CAD build for the part. Positions are in the model's coordinates, mm. A direction names the side the tool comes from. Round coordinates to 2 decimals unless told otherwise and drop trailing zeros. Write each loop counter-clockwise with the first axis right and the second up, starting at its lowest first coordinate (ties: lowest second). Pieces come first, ordered by that corner, then holes. Notation, with made-up numbers: (40, -25) - (82, -25) arc R12 ccw to (82, -9) - close; hole circle Ø5 at (65, 13). An arc over 180 degrees is marked (long way). Put each result on its own line as item: value. Start each with the question number.
Item 1: Mould opens along Z. For faces 1 (the flat face through (30, 1, -150)), 2 (the flat face through (-25.4, 1.48, -132.08)), 3 (the cylindrical face through (-0.88, 1.48, -122.9)) say: released by +Z, released by -Z, zero draft, split by the parting line, or undercut.
Item 2: Cut at A-A (z = -157.5). Give the cut face in (x, y), and give its area (3 significant figures).
Item 3: 3-axis set-ups, long thin cutter, end or side, ignore diameter. For faces 4 (the cylindrical face through (22.39, 1.48, -136.02)), 5 (the flat face through (-15, 1, -126.088)), 6 (the flat face through (15, 1, -126.088)): which of +Z, -Z, +X, -X, +Y, -Y reach the whole face in a straight line?
Item 4: Drill centre lines: line 1 (X direction, y = 1, z = -157.5); line 2 (X direction, y = 1.85, z = -136); line 3 (Z direction, x = -14, y = 0.8). Where is each one in solid material? Low to high. Write a range as from..to.
Item 5: Pin check, flat tips, straight feed: pin 1 Ø1 at (y, z) = (1.5, -128.5) entering from -X; pin 2 Ø4 at (x, z) = (14.1, -141.03) entering from +Y; pin 3 Ø0.9 at (y, z) = (2, -121.5) entering from -X; pin 4 Ø1.5 at (x, y) = (-14, 2) entering from +Z. Stop position of each tip, or through.
Item 6: Cut at B-B (x = 0). Give the cut face in (y, z).
Item 7: Cut at C-C (z = -141.5). Give the cut face in (x, y).
Item 8: Cut at D-D (y = 0.45). Count the separate pieces of the cut face and the enclosed holes in it, and give its area (3 significant figures).
```python
from build123d import *

# Parameters (mm, degrees)
SKETCH_1_R      = 1.45
EXTRUDE_1_DEPTH = 3
FILLET_1_R      = 3


with BuildPart() as part:
    # 草图1 → 凸台-拉伸1 (new body)
    with BuildSketch(Plane(origin=(0, 0, 0), x_dir=(1, 0, 0), z_dir=(0, 1, 0))):
        Polygon((30, 165), (-30, 165), (-30, 137.678611726), (-20.478927243, 126.087702635), (-7.5, 126.087702635), (-7.5, 116.748929431), (7.5, 116.748929431), (7.5, 126.087702635), (20.478927243, 126.087702635), (30, 137.678611726), align=None)
        with Locations(Location((0, 157.5, 0), (0, 0, 270))):
            Circle(SKETCH_1_R, mode=Mode.SUBTRACT)
        with Locations(Location((-15, 157.5, 0), (0, 0, 270))):
            Circle(SKETCH_1_R, mode=Mode.SUBTRACT)
        with Locations(Location((-14.103099985, 141.030854536, 0), (0, 0, 270))):
            Circle(SKETCH_1_R, mode=Mode.SUBTRACT)
        with Locations(Location((-21.830372712, 134.683472697, 0), (0, 0, 270))):
            Circle(SKETCH_1_R, mode=Mode.SUBTRACT)
        with Locations(Location((21.830372712, 134.683472697, 0), (0, 0, 90))):
            Circle(SKETCH_1_R, mode=Mode.SUBTRACT)
        with Locations(Location((14.103099985, 141.030854536, 0), (0, 0, 90))):
            Circle(SKETCH_1_R, mode=Mode.SUBTRACT)
        with Locations(Location((15, 157.5, 0), (0, 0, 90))):
            Circle(SKETCH_1_R, mode=Mode.SUBTRACT)
        with Locations(Location((0, 131.748929431, 0), (0, 0, 270))):
            Circle(SKETCH_1_R, mode=Mode.SUBTRACT)
        with Locations(Location((0, 121.748929431, 0), (0, 0, 270))):
            Circle(SKETCH_1_R, mode=Mode.SUBTRACT)
    extrude(amount=EXTRUDE_1_DEPTH)

    # 圆角1
    fillet_1_edges = [part.edges().sort_by_distance(p)[0] for p in [
        (-30, 1.5, -165),
        (30, 1.5, -165),
        (30, 1.5, -137.678611726),
        (20.478927243, 1.5, -126.087702635),
        (7.5, 1.5, -126.087702635),
        (7.5, 1.5, -116.748929431),
        (-7.5, 1.5, -116.748929431),
        (-7.5, 1.5, -126.087702635),
        (-20.478927243, 1.5, -126.087702635),
        (-30, 1.5, -137.678611726),
    ]]
    fillet(fillet_1_edges, radius=FILLET_1_R)


solid = part.part
```
Output values:
1. face 1: zero draft
1. face 2: released by +Z
1. face 3: undercut
2. outline: (-30, 0) - (-16.45, 0) - (-16.45, 3) - (-30, 3) - close; (-13.55, 0) - (-1.45, 0) - (-1.45, 3) - (-13.55, 3) - close; (1.45, 0) - (13.55, 0) - (13.55, 3) - (1.45, 3) - close; (16.45, 0) - (30, 0) - (30, 3) - (16.45, 3) - close
2. area: 154 mm2
3. face 4: +Y, -Y
3. face 5: +Z, -X, +Y, -Y
3. face 6: +Z, +X, +Y, -Y
4. line 1: -30..-16.45, -13.55..-1.45, 1.45..13.55, 16.45..30
4. line 2: -28.62..-22.44, -21.22..21.22, 22.44..28.62
4. line 3: -165..-158.55, -156.45..-142.48, -139.58..-126.09
5. pin 1: x = -22.87
5. pin 2: y = 3
5. pin 3: x = -7.5
5. pin 4: z = -126.09
6. outline: (0, -165) - (3, -165) - (3, -158.95) - (0, -158.95) - close; (0, -156.05) - (3, -156.05) - (3, -133.2) - (0, -133.2) - close; (0, -130.3) - (3, -130.3) - (3, -123.2) - (0, -123.2) - close; (0, -120.3) - (3, -120.3) - (3, -116.75) - (0, -116.75) - close
7. outline: (-30, 0) - (-15.48, 0) - (-15.48, 3) - (-30, 3) - close; (-12.73, 0) - (12.73, 0) - (12.73, 3) - (-12.73, 3) - close; (15.48, 0) - (30, 0) - (30, 3) - (15.48, 3) - close
8. separate pieces: 1
8. enclosed holes: 9
8. area: 2,300 mm2
